For this review, take the finished solid that the model builds, in its own axes (mm). A direction names the side the tool comes from. Give positions to 0.01 mm unless a question says otherwise; leave off trailing zeros. Write each loop counter-clockwise with the first axis right and the second up, starting at its lowest first coordinate (ties: lowest second). Pieces come first, ordered by that corner, then holes. Notation, with made-up numbers: (42.5, 36) -> (86.5, 36) arc R23 cw to (86.5, 54) -> close; hole circle Ø2 at (78, 27). An arc over 180 degrees is marked (long way). Write item = value, one per line.
Autodesk Inventor part; units mm, degrees
ref_plane "YZ Plane" through (0, 0, 0) normal (1, 0, 0) x (0, 1, 0)
ref_plane "XY Plane" through (0, 0, 0) normal (0, 0, 1) x (1, 0, 0)
sketch "Эскиз1" plane through (0, 0, 0) normal (0, 0, 1) x (1, 0, 0)
  line L0 (-7.8, 4.75) -> (0, 4.75)
  line L1 (0, 4.75) -> (0, 5)
  line L2 (0, 5) -> (6.5, 5)
  line L3 (6.5, 5) -> (6.5, 5.3)
  line L4 (6.5, 5.3) -> (5.2876, 6)
  line L5 (5.2876, 6) -> (-2.1, 6)
  line L6 (-2.1, 6) -> (-2.1, 7.5)
  line L7 (-2.1, 7.5) -> (-3.1, 7.5)
  line L8 (-3.1, 7.5) -> (-3.1, 6.5)
  line L9 (-3.1, 6.5) -> (-7.8, 6.5)
  line L10 (-6.6244, 0) -> (6.6244, 0) construction
  line L11 (-8.1, 6.2) -> (-8.1, 5.05)
  line L12 (-7.8, 6.5) -> (-8.1, 6.2)
  line L13 (-8.1, 5.05) -> (-7.8, 4.75)
  point P0 (0, 0)
  point P1 (-8.1, 6.5)
  point P2 (-8.1, 4.75)
  point P3 (0, 0)
  dimension "d2" = 12
  dimension "d3" = 15
  dimension "d8" = 13
  dimension "d9" = 1
  dimension "d10" = 0.3
  dimension "d11" = 120
  dimension "d12" = 6.5
  dimension "d14" = 0.3
  dimension "d15" = 0.3
  dimension "d16" = 0.3
  dimension "d17" = 0.3
  dimension "d18" = 9.5
  dimension "d19" = 5
  dimension "d20" = 1
  dimension "d21" = 8.6
  dimension "inside" = 10
revolve "Вращение1" add sketch "Эскиз1" angle 360 about axis through (-6.6244, 0, 0) along (1, 0, 0)
thread "Резьба1"
thread "Резьба2"
ref_plane "РабПлоскость1" through (1.5938, 6, 0) normal (0, 1, 0) x (-1, 0, 0)
sketch "Эскиз2" plane through (1.5938, 6, 0) normal (0, 1, 0) x (-1, 0, 0)
  line L0 (3.6938, 5) -> (-6.3062, 5)
  line L1 (-6.3062, 5) -> (-6.3062, -5)
  line L2 (-6.3062, -5) -> (3.6938, -5)
  line L3 (3.6938, -5) -> (3.6938, 5)
  line L4 (3.6938, 7.5) -> (3.6938, -7.5)
  point P0 (1.5938, 0)
  point P1 (-6.3062, 0)
  point P2 (3.6938, 0)
  dimension "d28" = 10
  dimension "d29" = 10
extrude "Выдавливание1" cut sketch "Эскиз2" against normal blind 0.5
sketch "Эскиз3" plane through (1.5938, 6, 0) normal (0, 1, 0) x (-1, 0, 0)
  line L0 (4.6938, 7.5) -> (4.6938, -7.5)
  line L1 (4.6938, -4) -> (12.6938, -4)
  line L2 (12.6938, -4) -> (12.6938, 4)
  line L3 (12.6938, 4) -> (4.6938, 4)
  line L4 (4.6938, 4) -> (4.6938, -4)
  point P0 (1.5938, 0)
  point P1 (4.6938, 0)
  dimension "d32" = 8
  dimension "d33" = 8
extrude "Выдавливание2" cut sketch "Эскиз3" along normal blind 0.5
mirror "Зеркальное отражение1" about plane through (0, 0, 0) normal (0, 1, 0) of "Выдавливание1", "Выдавливание2"
equation "\"d29\" = d28"
properties part number "корпус разъема" material "Сталь, нержавеющая, полированная"
(1) Take a section at C-C (x = -1.5). Write out the cut boundary in (y, z).
Answers below:
outline = (-5.5, -2.4) arc R6 ccw to (5.5, -2.4) -> (5.5, 2.4) arc R6 ccw to (-5.5, 2.4) -> close; hole circle Ø9.5 at (0, 0)
(2) Take a section at A-A (y = 0). Write out the cut boundary in (x, z).
Answers below:
outline = (-8.1, -6.2) -> (-7.8, -6.5) -> (-3.1, -6.5) -> (-3.1, -7.5) -> (-2.1, -7.5) -> (-2.1, -6) -> (5.29, -6) -> (6.5, -5.3) -> (6.5, -5) -> (0, -5) -> (0, -4.75) -> (-7.8, -4.75) -> (-8.1, -5.05) -> close; (-8.1, 5.05) -> (-7.8, 4.75) -> (0, 4.75) -> (0, 5) -> (6.5, 5) -> (6.5, 5.3) -> (5.29, 6) -> (-2.1, 6) -> (-2.1, 7.5) -> (-3.1, 7.5) -> (-3.1, 6.5) -> (-7.8, 6.5) -> (-8.1, 6.2) -> close
(3) For pin 1 (5.5 mm diameter, centred on x = -7, z = 0.5, fed in from -Y); pin 2 (2 mm diameter, centred on x = -1.5, z = 5, fed in from -Y); pin 3 (3 mm diameter, centred on y = 0.5, z = 4.5, fed in from -X); pin 4 (4 mm diameter, centred on x = 3.5, z = 1, fed in from +Y), all flat-tipped, find the tip position at first contact; note any pin that passes through.
Answers below:
pin_1 = -6
pin_2 = -6.21
pin_3 = -8.1
pin_4 = 5.5
(4) Take a section at B-B (z = 0). Write out the cut boundary in (x, y).
Answers below:
outline = (-8.1, -6) -> (-3.1, -6) -> (-3.1, -7.5) -> (-2.1, -7.5) -> (-2.1, -5.5) -> (6.15, -5.5) -> (6.5, -5.3) -> (6.5, -5) -> (0, -5) -> (0, -4.75) -> (-7.8, -4.75) -> (-8.1, -5.05) -> close; (-8.1, 5.05) -> (-7.8, 4.75) -> (0, 4.75) -> (0, 5) -> (6.5, 5) -> (6.5, 5.3) -> (6.15, 5.5) -> (-2.1, 5.5) -> (-2.1, 7.5) -> (-3.1, 7.5) -> (-3.1, 6) -> (-8.1, 6) -> close
(5) Take a section at D-D (x = 5). Write out the cut boundary in (y, z), plus the area to 3 significant figures.
Answers below:
outline = (-5.5, -2.4) arc R6 ccw to (5.5, -2.4) -> (5.5, 2.4) arc R6 ccw to (-5.5, 2.4) -> close; hole circle Ø10 at (0, 0)
area = 31.3 mm^2
(6) Tool access review of faces 1 (the face through (-3.1, 6.15, -0.04)), 2 (the face through (-6, 6, 0)), 3 (the face through (3.3, -1.08, -4.88)), 4 (the face through (2, -5.5, 0)): name each direction out of +Z, -Z, +X, -X, +Y, -Y from which nothing blocks a thin tool from reaching the whole face with its end or side.
Answers below:
face_1 = -X
face_2 = +Z, -Z, -X, +Y
face_3 = +X
face_4 = +Z, -Z, +X, -Y
(7) The part is to be moulded in two halves that separate along Y. For faces 5 (the face through (-6, -6, 0)), 6 (the face through (-2.1, 6, 1)), 7 (the face through (-3.845, 2.192, -4.214)), 8 (the face through (-7.98, 0.12, 6.32)), say which applies: released by +Y, released by -Y, zero draft, split by the parting line, or undercut.
Answers below:
face_5 = released by -Y
face_6 = zero draft
face_7 = undercut
face_8 = split by the parting line
(8) To check wall thickness, follow probe 1 along Z at (x, y) = (-2.25, 0); probe 2 along Z at (x, y) = (5, 0); probe 3 along X at (y, z) = (-6.25, 0). State the ranges of each line that lie inside material, in increasing order.
Answers below:
probe_1 = -7.5 to -4.75, 4.75 to 7.5
probe_2 = -6 to -5, 5 to 6
probe_3 = -3.1 to -2.1
